from build123d import *

# Parameters (mm, degrees)
SKETCH001_W     = 304
SKETCH001_H     = 114
SKETCH001_W_2   = 287
SKETCH001_H_2   = 97
PAD_DEPTH       = 16
FILLET_R        = 2
FILLET001_R     = 2
FILLET002_R     = 2
FILLET003_R     = 2
FILLET004_R     = 5
FILLET005_R     = 5
FILLET006_R     = 5
FILLET007_R     = 5
SKETCH002_W     = 297
SKETCH002_H     = 107
POCKET_DEPTH    = 7
FILLET008_R     = 3
FILLET009_R     = 3
FILLET010_R     = 3
FILLET011_R     = 3
SKETCH003_W     = 80
SKETCH003_H     = 5
POCKET001_DEPTH = 3.5
SKETCH004_W     = 5
SKETCH004_H     = 32.5
POCKET002_DEPTH = 3.5
FILLET012_R     = 5
FILLET013_R     = 1
FILLET014_R     = 1
FILLET015_R     = 1
FILLET016_R     = 1
FILLET017_R     = 1
FILLET018_R     = 1
FILLET019_R     = 1
FILLET020_R     = 1
FILLET021_R     = 1
FILLET022_R     = 1
FILLET023_R     = 1
FILLET024_R     = 1
FILLET025_R     = 1
FILLET026_R     = 1
FILLET027_R     = 1
FILLET028_R     = 1
FILLET029_R     = 1
FILLET030_R     = 1
FILLET031_R     = 1
FILLET032_R     = 1
FILLET033_R     = 1
FILLET034_R     = 1
FILLET035_R     = 1
FILLET036_R     = 1
FILLET037_R     = 1
FILLET038_R     = 1
FILLET039_R     = 1
FILLET040_R     = 1
FILLET041_R     = 1
FILLET042_R     = 1
FILLET043_R     = 1
FILLET044_R     = 1
FILLET045_R     = 1
FILLET046_R     = 1
FILLET047_R     = 1
FILLET048_R     = 1
FILLET049_R     = 1
FILLET050_R     = 1
FILLET051_R     = 1
FILLET052_R     = 1
FILLET053_R     = 1


with BuildPart() as part:
    # Sketch001 → Pad (new body)
    with BuildSketch(Plane.XY):
        Rectangle(SKETCH001_W, SKETCH001_H)
        Rectangle(SKETCH001_W_2, SKETCH001_H_2, mode=Mode.SUBTRACT)
    extrude(amount=PAD_DEPTH)

    # Fillet
    fillet_edges = [part.edges().sort_by_distance(p)[0] for p in [
        (-143.5, -48.5, 8),
    ]]
    fillet(fillet_edges, radius=FILLET_R)

    # Fillet001
    fillet001_edges = [part.edges().sort_by_distance(p)[0] for p in [
        (143.5, -48.5, 8),
    ]]
    fillet(fillet001_edges, radius=FILLET001_R)

    # Fillet002
    fillet002_edges = [part.edges().sort_by_distance(p)[0] for p in [
        (-143.5, 48.5, 8),
    ]]
    fillet(fillet002_edges, radius=FILLET002_R)

    # Fillet003
    fillet003_edges = [part.edges().sort_by_distance(p)[0] for p in [
        (143.5, 48.5, 8),
    ]]
    fillet(fillet003_edges, radius=FILLET003_R)

    # Fillet004
    fillet004_edges = [part.edges().sort_by_distance(p)[0] for p in [
        (-152, -57, 8),
    ]]
    fillet(fillet004_edges, radius=FILLET004_R)

    # Fillet005
    fillet005_edges = [part.edges().sort_by_distance(p)[0] for p in [
        (-152, 57, 8),
    ]]
    fillet(fillet005_edges, radius=FILLET005_R)

    # Fillet006
    fillet006_edges = [part.edges().sort_by_distance(p)[0] for p in [
        (152, -57, 8),
    ]]
    fillet(fillet006_edges, radius=FILLET006_R)

    # Fillet007
    fillet007_edges = [part.edges().sort_by_distance(p)[0] for p in [
        (152, 57, 8),
    ]]
    fillet(fillet007_edges, radius=FILLET007_R)

    # Sketch002 (on Face1 of Fillet007) → Pocket (cut)
    with BuildSketch(Plane(origin=(0, 0, 0), x_dir=(1, 0, 0), z_dir=(0, 0, -1))):
        Rectangle(SKETCH002_W, SKETCH002_H)
    extrude(amount=-POCKET_DEPTH, mode=Mode.SUBTRACT)

    # Fillet008
    fillet008_edges = [part.edges().sort_by_distance(p)[0] for p in [
        (-148.5, -53.5, 3.5),
    ]]
    fillet(fillet008_edges, radius=FILLET008_R)

    # Fillet009
    fillet009_edges = [part.edges().sort_by_distance(p)[0] for p in [
        (-148.5, 53.5, 3.5),
    ]]
    fillet(fillet009_edges, radius=FILLET009_R)

    # Fillet010
    fillet010_edges = [part.edges().sort_by_distance(p)[0] for p in [
        (148.5, 53.5, 3.5),
    ]]
    fillet(fillet010_edges, radius=FILLET010_R)

    # Fillet011
    fillet011_edges = [part.edges().sort_by_distance(p)[0] for p in [
        (148.5, -53.5, 3.5),
    ]]
    fillet(fillet011_edges, radius=FILLET011_R)

    # Sketch003 (on Face18 of Fillet011) → Pocket001 (cut)
    with BuildSketch(Plane(origin=(0, 0, 7), x_dir=(1, 0, 0), z_dir=(0, 0, -1))):
        with Locations((0, 51)):
            Rectangle(SKETCH003_W, SKETCH003_H)
        with Locations((0, -51)):
            Rectangle(SKETCH003_W, SKETCH003_H)
        with Locations((-95, 51)):
            Rectangle(SKETCH003_W, SKETCH003_H)
        with Locations((95, 51)):
            Rectangle(SKETCH003_W, SKETCH003_H)
        with Locations((95, -51)):
            Rectangle(SKETCH003_W, SKETCH003_H)
        with Locations((-95, -51)):
            Rectangle(SKETCH003_W, SKETCH003_H)
    extrude(amount=-POCKET001_DEPTH, mode=Mode.SUBTRACT)

    # Sketch004 (on Face18 of Pocket001) → Pocket002 (cut)
    with BuildSketch(Plane(origin=(0, 0, 7), x_dir=(1, 0, 0), z_dir=(0, 0, -1))):
        with Locations((-146, 23.75)):
            Rectangle(SKETCH004_W, SKETCH004_H)
        with Locations((146, 23.75)):
            Rectangle(SKETCH004_W, SKETCH004_H)
        with Locations((146, -23.75)):
            Rectangle(SKETCH004_W, SKETCH004_H)
        with Locations((-146, -23.75)):
            Rectangle(SKETCH004_W, SKETCH004_H)
    extrude(amount=-POCKET002_DEPTH, mode=Mode.SUBTRACT)

    # Fillet012
    fillet012_edges = [part.edges().sort_by_distance(p)[0] for p in [
        (-150.535534, 55.535534, 16),
    ]]
    fillet(fillet012_edges, radius=FILLET012_R)

    # Fillet013
    fillet013_edges = [part.edges().sort_by_distance(p)[0] for p in [
        (-150.535534, 55.535534, 0),
    ]]
    fillet(fillet013_edges, radius=FILLET013_R)

    # Fillet014
    fillet014_edges = [part.edges().sort_by_distance(p)[0] for p in [
        (-135, -48.5, 8.75),
    ]]
    fillet(fillet014_edges, radius=FILLET014_R)

    # Fillet015
    fillet015_edges = [part.edges().sort_by_distance(p)[0] for p in [
        (-143.5, -40, 8.75),
    ]]
    fillet(fillet015_edges, radius=FILLET015_R)

    # Fillet016
    fillet016_edges = [part.edges().sort_by_distance(p)[0] for p in [
        (-135, -53.5, 8.75),
    ]]
    fillet(fillet016_edges, radius=FILLET016_R)

    # Fillet017
    fillet017_edges = [part.edges().sort_by_distance(p)[0] for p in [
        (-148.5, -40, 8.75),
    ]]
    fillet(fillet017_edges, radius=FILLET017_R)

    # Fillet018
    fillet018_edges = [part.edges().sort_by_distance(p)[0] for p in [
        (-40, -53.5, 8.75),
    ]]
    fillet(fillet018_edges, radius=FILLET018_R)

    # Fillet019
    fillet019_edges = [part.edges().sort_by_distance(p)[0] for p in [
        (-40, -48.5, 8.75),
    ]]
    fillet(fillet019_edges, radius=FILLET019_R)

    # Fillet020
    fillet020_edges = [part.edges().sort_by_distance(p)[0] for p in [
        (-55, -48.5, 8.75),
    ]]
    fillet(fillet020_edges, radius=FILLET020_R)

    # Fillet021
    fillet021_edges = [part.edges().sort_by_distance(p)[0] for p in [
        (-55, -53.5, 8.75),
    ]]
    fillet(fillet021_edges, radius=FILLET021_R)

    # Fillet022
    fillet022_edges = [part.edges().sort_by_distance(p)[0] for p in [
        (40, -48.5, 8.75),
    ]]
    fillet(fillet022_edges, radius=FILLET022_R)

    # Fillet023
    fillet023_edges = [part.edges().sort_by_distance(p)[0] for p in [
        (40, -53.5, 8.75),
    ]]
    fillet(fillet023_edges, radius=FILLET023_R)

    # Fillet024
    fillet024_edges = [part.edges().sort_by_distance(p)[0] for p in [
        (55, -48.5, 8.75),
    ]]
    fillet(fillet024_edges, radius=FILLET024_R)

    # Fillet025
    fillet025_edges = [part.edges().sort_by_distance(p)[0] for p in [
        (55, -53.5, 8.75),
    ]]
    fillet(fillet025_edges, radius=FILLET025_R)

    # Fillet026
    fillet026_edges = [part.edges().sort_by_distance(p)[0] for p in [
        (148.5, -40, 8.75),
    ]]
    fillet(fillet026_edges, radius=FILLET026_R)

    # Fillet027
    fillet027_edges = [part.edges().sort_by_distance(p)[0] for p in [
        (143.5, -40, 8.75),
    ]]
    fillet(fillet027_edges, radius=FILLET027_R)

    # Fillet028
    fillet028_edges = [part.edges().sort_by_distance(p)[0] for p in [
        (135, -48.5, 8.75),
    ]]
    fillet(fillet028_edges, radius=FILLET028_R)

    # Fillet029
    fillet029_edges = [part.edges().sort_by_distance(p)[0] for p in [
        (135, -53.5, 8.75),
    ]]
    fillet(fillet029_edges, radius=FILLET029_R)

    # Fillet030
    fillet030_edges = [part.edges().sort_by_distance(p)[0] for p in [
        (148.5, 7.5, 8.75),
    ]]
    fillet(fillet030_edges, radius=FILLET030_R)

    # Fillet031
    fillet031_edges = [part.edges().sort_by_distance(p)[0] for p in [
        (143.5, 7.5, 8.75),
    ]]
    fillet(fillet031_edges, radius=FILLET031_R)

    # Fillet032
    fillet032_edges = [part.edges().sort_by_distance(p)[0] for p in [
        (143.5, -7.5, 8.75),
    ]]
    fillet(fillet032_edges, radius=FILLET032_R)

    # Fillet033
    fillet033_edges = [part.edges().sort_by_distance(p)[0] for p in [
        (148.5, -7.5, 8.75),
    ]]
    fillet(fillet033_edges, radius=FILLET033_R)

    # Fillet034
    fillet034_edges = [part.edges().sort_by_distance(p)[0] for p in [
        (148.5, 40, 8.75),
    ]]
    fillet(fillet034_edges, radius=FILLET034_R)

    # Fillet035
    fillet035_edges = [part.edges().sort_by_distance(p)[0] for p in [
        (143.5, 40, 8.75),
    ]]
    fillet(fillet035_edges, radius=FILLET035_R)

    # Fillet036
    fillet036_edges = [part.edges().sort_by_distance(p)[0] for p in [
        (135, 48.5, 8.75),
    ]]
    fillet(fillet036_edges, radius=FILLET036_R)

    # Fillet037
    fillet037_edges = [part.edges().sort_by_distance(p)[0] for p in [
        (135, 53.5, 8.75),
    ]]
    fillet(fillet037_edges, radius=FILLET037_R)

    # Fillet038
    fillet038_edges = [part.edges().sort_by_distance(p)[0] for p in [
        (40, 53.5, 8.75),
    ]]
    fillet(fillet038_edges, radius=FILLET038_R)

    # Fillet039
    fillet039_edges = [part.edges().sort_by_distance(p)[0] for p in [
        (40, 48.5, 8.75),
    ]]
    fillet(fillet039_edges, radius=FILLET039_R)

    # Fillet040
    fillet040_edges = [part.edges().sort_by_distance(p)[0] for p in [
        (55, 48.5, 8.75),
    ]]
    fillet(fillet040_edges, radius=FILLET040_R)

    # Fillet041
    fillet041_edges = [part.edges().sort_by_distance(p)[0] for p in [
        (55, 53.5, 8.75),
    ]]
    fillet(fillet041_edges, radius=FILLET041_R)

    # Fillet042
    fillet042_edges = [part.edges().sort_by_distance(p)[0] for p in [
        (-40, 53.5, 8.75),
    ]]
    fillet(fillet042_edges, radius=FILLET042_R)

    # Fillet043
    fillet043_edges = [part.edges().sort_by_distance(p)[0] for p in [
        (-40, 48.5, 8.75),
    ]]
    fillet(fillet043_edges, radius=FILLET043_R)

    # Fillet044
    fillet044_edges = [part.edges().sort_by_distance(p)[0] for p in [
        (-55, 53.5, 8.75),
    ]]
    fillet(fillet044_edges, radius=FILLET044_R)

    # Fillet045
    fillet045_edges = [part.edges().sort_by_distance(p)[0] for p in [
        (-55, 48.5, 8.75),
    ]]
    fillet(fillet045_edges, radius=FILLET045_R)

    # Fillet046
    fillet046_edges = [part.edges().sort_by_distance(p)[0] for p in [
        (-135, 53.5, 8.75),
    ]]
    fillet(fillet046_edges, radius=FILLET046_R)

    # Fillet047
    fillet047_edges = [part.edges().sort_by_distance(p)[0] for p in [
        (-135, 48.5, 8.75),
    ]]
    fillet(fillet047_edges, radius=FILLET047_R)

    # Fillet048
    fillet048_edges = [part.edges().sort_by_distance(p)[0] for p in [
        (-143.5, 40, 8.75),
    ]]
    fillet(fillet048_edges, radius=FILLET048_R)

    # Fillet049
    fillet049_edges = [part.edges().sort_by_distance(p)[0] for p in [
        (-148.5, 40, 8.75),
    ]]
    fillet(fillet049_edges, radius=FILLET049_R)

    # Fillet050
    fillet050_edges = [part.edges().sort_by_distance(p)[0] for p in [
        (-148.5, 7.5, 8.75),
    ]]
    fillet(fillet050_edges, radius=FILLET050_R)

    # Fillet051
    fillet051_edges = [part.edges().sort_by_distance(p)[0] for p in [
        (-143.5, 7.5, 8.75),
    ]]
    fillet(fillet051_edges, radius=FILLET051_R)

    # Fillet052
    fillet052_edges = [part.edges().sort_by_distance(p)[0] for p in [
        (-148.5, -7.5, 8.75),
    ]]
    fillet(fillet052_edges, radius=FILLET052_R)

    # Fillet053
    fillet053_edges = [part.edges().sort_by_distance(p)[0] for p in [
        (-143.5, -7.5, 8.75),
    ]]
    fillet(fillet053_edges, radius=FILLET053_R)


solid = part.part
Source: CAD feature listing. Evaluate the final solid. Frame: model axes, mm. A direction names the side the tool comes from. Round coordinates to 2 decimals unless told otherwise and drop trailing zeros. Loops run counter-clockwise (first coordinate to the right, second up) from the corner with the lowest first, then second, coordinate; pieces in that order, holes last.
Q1. Ray query, line 1 (Y direction, x = 37, z = 7); line 2 (Y direction, x = -111, z = 11.5); line 3 (X direction, y = 44.5, z = 3). Return the intervals inside material, ascending.
Q2. First-contact query: P1, Ø4, axis at x = -81, y = -50.5, coming from the -Z side; P2, Ø5.5, axis at x = -48.5, y = -50, coming from the -Z side; P3, Ø1, axis at y = -36, z = 13.5, coming from the +X side. Flat tips, straight axial feed; report the tip coordinate or a pass-through.
Q3. Section B-B, the plane y = 28. Return loops of the section in (x, z), plus the area to 3 significant figures.
Q4. Section A-A, the plane x = -44. Return loops of the section in (y, z), plus the area to 3 significant figures.
Q5. Section C-C, the plane z = 4. Return loops of the section in (x, y), plus the area to 3 significant figures.
Q6. Access query for faces 4 (the face through (-146, -24, 10.5)), 5 (the face through (143.5, -1, 12)), 6 (the face through (-1, 54, 0)). Directions: +Z, -Z, +X, -X, +Y, -Y. A direction counts if a zero-diameter tool reaches every point of the face in a straight line with its end or side. Return the directions, or none.
Q7. Mould query, pull axis Y, two halves, no side actions, for faces 1 (the face through (150, -56, 6)), 2 (the face through (-96, -51, 10.5)), 3 (the face through (-1, 50, 16)). Classes: pulls with the +Y half, pulls with the -Y half, needs draft (parallel to the pull), parting line crosses it, or undercut.
Solutions:
1. line 1: y = -57 to -53.5, 53.5 to 57
1. line 2: y = -56.97 to -48.5, 48.5 to 56.97
1. line 3: x = -152 to -148.5, 148.5 to 152
2. P1: stops at z = 10.5
2. P2: stops at z = 7
2. P3: stops at x = 151.58
3. outline: (-152, 1) arc R1 ccw to (-151, 0) - (-148.5, 0) - (-148.5, 10.5) - (-143.5, 10.5) - (-143.5, 16) - (-147, 16) arc R5 ccw to (-152, 11) - close; (143.5, 10.5) - (148.5, 10.5) - (148.5, 0) - (151, 0) arc R1 ccw to (152, 1) - (152, 11) arc R5 ccw to (147, 16) - (143.5, 16) - close
3. area: 156 mm2
4. outline: (-57, 1) arc R1 ccw to (-56, 0) - (-53.5, 0) - (-53.5, 7) - (-48.5, 7) - (-48.5, 16) - (-52, 16) arc R5 ccw to (-57, 11) - close; (48.5, 7) - (53.5, 7) - (53.5, 0) - (56, 0) arc R1 ccw to (57, 1) - (57, 11) arc R5 ccw to (52, 16) - (48.5, 16) - close
4. area: 191 mm2
5. outline: (-152, -52) arc R5 ccw to (-147, -57) - (147, -57) arc R5 ccw to (152, -52) - (152, 52) arc R5 ccw to (147, 57) - (-147, 57) arc R5 ccw to (-152, 52) - close; hole (-148.5, -50.5) arc R3 ccw to (-145.5, -53.5) - (145.5, -53.5) arc R3 ccw to (148.5, -50.5) - (148.5, 50.5) arc R3 ccw to (145.5, 53.5) - (-145.5, 53.5) arc R3 ccw to (-148.5, 50.5) - close
5. area: 2,860 mm2
6. face 4: -Z
6. face 5: +Z, -Z
6. face 6: -Z, +X, -X, +Y, -Y
7. face 1: pulls with the -Y half
7. face 2: undercut
7. face 3: needs draft
